Source: CAD feature listing. Evaluate the final solid. Frame: model axes, mm. A direction names the side the tool comes from. Round coordinates to 2 decimals unless told otherwise and drop trailing zeros. Order: outer loops, then holes, each group sorted by start corner. A loop starts at its lowest first (then second) coordinate and runs counter-clockwise, first axis right, second up. Notation, with made-up numbers: (14.25, -0.5) - (23.25, -0.5) arc R18 cw to (23.25, 27.5) - close; hole circle Ø5 at (-29, 70.25). An arc over 180 degrees is marked (long way). Return JSON: item names as keys, results as strings. Group by question number.
1) Mould query, pull axis Y, two halves, no side actions, for faces 1 (the cylindrical face through (-0.471, -44.147, 5.935)), 2 (the flat face through (43, -30.5, 4)), 3 (the flat face through (43, 30.5, 4)), 4 (the flat face through (-1, 1, 0)). Classes: pulls with the +Y half, pulls with the -Y half, needs draft (parallel to the pull), parting line crosses it, or undercut.
2) Ray query, line 1 (X direction, y = 27.5, z = 1.5); line 2 (Z direction, x = -42, y = 23.5); line 3 (X direction, y = -38.5, z = 1). Return the intervals inside material, ascending. Write a range as from..to.
3) Section A-A, the plane y = -11. Return loops of the section in (x, z), plus the area to 3 significant figures.
4) Section B-B, the plane x = 40.5. Return loops of the section in (y, z).
5) Section D-D, the plane y = 33.5. Return loops of the section in (x, z), plus the area to 3 significant figures.
6) Access query for faces 5 (the flat face through (-43, -30.5, 4)), 6 (the flat face through (30.5, -43, 4)), 7 (the flat face through (-30.5, 43, 4)), 8 (the flat face through (-54, 0, 6)), 9 (the flat face through (30.5, 43, 4)). Directions: +Z, -Z, +X, -X, +Y, -Y. A direction counts if a zero-diameter tool reaches every point of the face in a straight line with its end or side. Return the directions, or none.
7) Section C-C, the plane z = 10.5. Return loops of the section in (x, y) (3 decimals), plus the area to 3 significant figures.
8) Contact query for flat-ended pins moving along their axis: P1, Ø1.8, axis at y = -8, z = 3.5, coming from the -X side; P2, Ø6, axis at x = -4.5, z = 2, coming from the -Y side; P3, Ø4, axis at x = 31, y = 34.5, coming from the -Z side; P4, Ø2.5, axis at x = -37.5, z = 5.5, coming from the +Y side. Output: stop coordinate, or through.
```python
from build123d import *

# Parameters (mm, degrees)
F0_W             = 104.5
F0_H             = 104.5
F1_DEPTH         = 6
F2_W             = 110
F2_H             = 110
F2_W_2           = 104.5
F2_H_2           = 104.5
F3_DEPTH         = 2.4
F4_R             = 3.025
F5_DEPTH         = 10
F6_R             = 44.15
F6_R_2           = 3.025
F7_DEPTH         = 5
F8_R             = 3
F10_DEPTH        = 8.401
F10_COPIES_COUNT = 4


# Not quite as in the source:
# - a pattern or mirror of a feature is missing from the dataset's text; its kind, count and spacing are read off the source's solid


with BuildPart() as f1:
    # F0 (on Top) → F1 (new body)
    with BuildSketch(Plane.XY):
        Rectangle(F0_W, F0_H)
    extrude(amount=F1_DEPTH)

    # F2 (on face) → F3 (join)
    with BuildSketch(Plane.XY.offset(6)):
        Rectangle(F2_W, F2_H)
        Rectangle(F2_W_2, F2_H_2, mode=Mode.SUBTRACT)
        Rectangle(F2_W_2, F2_H_2)
    extrude(amount=F3_DEPTH)

    # F4 (on face) → F5 (join)
    with BuildSketch(Plane.XY.offset(8.4)):
        Circle(F4_R)
    extrude(amount=F5_DEPTH)

    # F6 (on face) → F7 (cut)
    with BuildSketch(Plane.XY.offset(8.4)):
        Circle(F6_R)
        Circle(F6_R_2, mode=Mode.SUBTRACT)
    extrude(amount=-F7_DEPTH, mode=Mode.SUBTRACT)

    # F8
    f8_edges = [f1.edges().sort_by_distance(p)[0] for p in [
        (-3.025, 0, 18.4),
    ]]
    fillet(f8_edges, radius=F8_R)

    # F9 (on face) → F10 (cut, through all)
    with BuildSketch(Plane.XY.offset(8.4)):
        with BuildLine():
            Line((-30.5, 31.9213486557), (-30.5, 55))
            Line((-30.5, 55), (-55, 55))
            Line((-55, 55), (-55, 30.5))
            Line((-55, 30.5), (-31.9213486557, 30.5))
            ThreePointArc((-31.9213486557, 30.5), (-31.2187643894, 31.2187643894), (-30.5, 31.9213486557))
        make_face()
        with BuildLine():
            Line((-30.5, 30.5), (-30.5, 31.9213486557))
            ThreePointArc((-30.5, 31.9213486557), (-31.2187643894, 31.2187643894), (-31.9213486557, 30.5))
            Line((-31.9213486557, 30.5), (-30.5, 30.5))
        make_face()
    f10 = extrude(amount=-F10_DEPTH, mode=Mode.SUBTRACT)

    # F10_copies: F10 ×4 about axis
    f10_copies_axis = Axis((0, 0, 0), (0, 0, 1))
    for i in range(1, F10_COPIES_COUNT):
        add(f10.rotate(f10_copies_axis, i * 360 / F10_COPIES_COUNT), mode=Mode.SUBTRACT)


solid = f1.part
```
Geometry check:
{
 "1": {"face 1": "undercut", "face 2": "pulls with the -Y half", "face 3": "pulls with the +Y half", "face 4": "needs draft"},
 "2": {"line 1": "-52.25..52.25", "line 2": "0..8.4", "line 3": "-30.5..30.5"},
 "3": {"outline": "(-55, 6) - (-52.25, 6) - (-52.25, 0) - (52.25, 0) - (52.25, 6) - (55, 6) - (55, 8.4) - (42.76, 8.4) - (42.76, 3.4) - (-42.76, 3.4) - (-42.76, 8.4) - (-55, 8.4) - close", "area": "463 mm2"},
 "4": {"outline": "(-30.5, 0) - (30.5, 0) - (30.5, 8.4) - (17.58, 8.4) - (17.58, 3.4) - (-17.58, 3.4) - (-17.58, 8.4) - (-30.5, 8.4) - close"},
 "5": {"outline": "(-30.5, 0) - (30.5, 0) - (30.5, 8.4) - (28.76, 8.4) - (28.76, 3.4) - (-28.76, 3.4) - (-28.76, 8.4) - (-30.5, 8.4) - close", "area": "225 mm2"},
 "6": {"face 5": "+Z, -Z, -X, -Y", "face 6": "+Z, -Z, +X, -Y", "face 7": "+Z, -Z, -X, +Y", "face 8": "-Z, -X, +Y, -Y", "face 9": "+Z, -Z, +X, +Y"},
 "7": {"outline": "circle Ø6.05 at (0, 0)", "area": "28.7 mm2"},
 "8": {"P1": "x = -52.25", "P2": "y = -52.25", "P3": "z = 0", "P4": "y = 30.5"}
}
